CAD build for the part. Positions are in the model's coordinates, mm. A direction names the side the tool comes from. Coordinates: 2 decimals unless noted, no trailing zeros. Loops run counter-clockwise (first coordinate to the right, second up) from the corner with the lowest first, then second, coordinate; pieces in that order, holes last. Notation, with made-up numbers: (36, -26.5) - (61, -26.5) arc R7 ccw to (61, -15.5) - close; hole circle Ø2 at (-27, 19.25). An arc over 180 degrees is marked (long way). Put each result on its own line as item: value.
Autodesk Inventor part; units mm, degrees
ref_plane "YZ Plane" through (0, 0, 0) normal (1, 0, 0) x (0, 1, 0)
ref_plane "XZ Plane" through (0, 0, 0) normal (0, 1, 0) x (-1, 0, 0)
sketch "Sketch1" plane through (0, 0, 0) normal (1, 0, 0) x (0, 1, 0)
  line L0 (11.5, 25) -> (-11.5, 25)
  line L1 (-11.5, 25) -> (-11.5, -25)
  line L2 (-11.5, -25) -> (11.5, -25)
  line L3 (11.5, -25) -> (11.5, 25)
  line L4 (11.5, 25) -> (-11.5, -25) construction
  line L5 (-11.5, 25) -> (11.5, -25) construction
  circle A0 centre (0, -30) radius 3.875
  line L6 (3.875, -30) -> (3.875, -25)
  line L7 (-3.875, -30) -> (-3.875, -25)
  line L8 (0, -45.65) -> (0, 36.775)
  circle A1 centre (0, -30) radius 2.1
  line L9 (-16.1, 0) -> (16.1, 0)
  circle A2 centre (-4.5, 0) radius 4
  line L10 (-4.5, 4) -> (-11.5, 4)
  line L11 (-4.5, -4) -> (-11.5, -4)
  point P0 (0, 0)
  point P1 (-11.5, 1.75)
  point P2 (-11.5, -4.25)
  point P3 (4, 25)
  point P4 (-4, 25)
  dimension "d0" = 50
  dimension "d1" = 23
  dimension "d4" = 7.75
  dimension "d5" = 5
  dimension "d6" = 4.2
  dimension "d11" = 8
  dimension "d12" = 7
extrude "Extrusion1" add sketch "Sketch1" along normal blind 2 contours L3 L9 L8 L0 | L8 L9 A2 L10 L1 L0 | L3 L2 L8 L9 | L8 L2 L1 L11 A2 L9 | L8 A0 L7 L2 | L2 L6 A0 L8 | L8 A1 A0 | A0 L8 A1
mirror "Mirror1" about plane through (0, 0, 0) normal (0, 0, 1) of "Extrusion1"
properties part number "pokrywa_baza"
Q1. Wall check: L1, parallel to Z at x = 1.05, y = 0 (3 decimals); L2, parallel to Z at x = 1.6, y = -10.25; L3, parallel to Y at x = 1.05, z = -30 (3 decimals). Give the ranges that are in metal, low to high. Write a range as from..to.
Determined:
L1: -33.875..-32.1, -27.9..27.9, 32.1..33.875
L2: -25..-4, 4..25
L3: -3.875..-2.1, 2.1..3.875
Q2. Mould opens along Y. For faces 6 (the cylindrical face through (1, -0.5, 0.1)), 7 (the cylindrical face through (0.99, -0.46, -27.95)), 8 (the flat face through (1, -8, 25)), 9 (the cylindrical face through (0.986, 0.969, 31.863)) say: +Y half, -Y half, draft (parallel to the pull), parting line (faces both ways), or undercut.
Determined:
face 6: -Y half
face 7: undercut
face 8: draft
face 9: undercut
Q3. Pin check, flat tips, straight feed: pin 1 Ø0.6 at (x, z) = (1.5, -28.5) entering from -Y (3 decimals); pin 2 Ø5 at (y, z) = (0, 30) entering from +X; pin 3 Ø0.6 at (x, y) = (0.5, -9) entering from -Z; pin 4 Ø3.5 at (y, z) = (0, -30) entering from -X. Stop position of each tip, or through.
Determined:
pin 1: y = -3.875
pin 2: x = 2
pin 3: z = -25
pin 4: through
Q4. Slice it at D-D, the plane z = 0. Give the cut face in (x, y), then the cut area to 3 significant figures.
Determined:
outline: (0, -0.5) - (2, -0.5) - (2, 11.5) - (0, 11.5) - close
area: 24.0 mm2
Q5. Slice it at B-B, the plane y = -1.5. Give the cut face in (x, z).
Determined:
outline: (0, -33.57) - (2, -33.57) - (2, -31.47) - (0, -31.47) - close; (0, -28.53) - (2, -28.53) - (2, -2.65) - (0, -2.65) - close; (0, 2.65) - (2, 2.65) - (2, 28.53) - (0, 28.53) - close; (0, 31.47) - (2, 31.47) - (2, 33.57) - (0, 33.57) - close
Q6. Slice it at C-C, the plane z = -29. Give the cut face in (x, y) (3 decimals), then the cut area to 3 significant figures.
Determined:
outline: (0, -3.875) - (2, -3.875) - (2, -1.847) - (0, -1.847) - close; (0, 1.847) - (2, 1.847) - (2, 3.875) - (0, 3.875) - close
area: 8.11 mm2
Q7. Tool access for faces 1 (the flat face through (1, -3.875, 27)), 2 (the flat face through (1, 8, 25)), 3 (the flat face through (1, -8, -25)), 4 (the flat face through (1, 8, -25)), 5 (the flat face through (1, -8, 4)): list every direction of +Z, -Z, +X, -X, +Y, -Y with a clear straight run to the whole face (end or side of a thin tool).
Determined:
face 1: +Z, +X, -X, -Y
face 2: +Z, +X, -X, +Y
face 3: -Z, +X, -X, -Y
face 4: -Z, +X, -X, +Y
face 5: +X, -X, -Y
Q8. Slice it at A-A, the plane x = 1.2. Give the cut face in (y, z) (3 decimals), then the cut area to 3 significant figures.
Determined:
outline: (-11.5, -25) - (-3.875, -25) - (-3.875, -30) arc R3.875 ccw to (3.875, -30) - (3.875, -25) - (11.5, -25) - (11.5, 25) - (3.875, 25) - (3.875, 30) arc R3.875 ccw to (-3.875, 30) - (-3.875, 25) - (-11.5, 25) - (-11.5, 4) - (-4.5, 4) arc R4 cw to (-4.5, -4) - (-11.5, -4) - close; hole circle Ø4.2 at (0, -30); hole circle Ø4.2 at (0, 30)
area: 1,170 mm2
